Could you check a few things on this model? Use its own coordinates, in mm. A direction names the side the tool comes from. Give positions to 0.01 mm unless a question says otherwise; leave off trailing zeros. Order: outer loops, then holes, each group sorted by start corner. A loop starts at its lowest first (then second) coordinate and runs counter-clockwise, first axis right, second up. Notation, with made-up numbers: M 50,-26 L 109,-26 A14 ccw 109,-14 Z; hole C -15.5,22.5 d1. An arc over 180 degrees is marked long. Use a Markdown table: item, result. Add a question column.
Item 1: If we mould it in two halves opening along Z, with no side actions, what happens to faces 1 (the face through (2.381, 4, -1)), 2 (the face through (3, 6, 2.496)), 3 (the face through (-0.732, 10.339, -2.326))? For each: released by +Z, released by -Z, zero draft, split by the parting line, or undercut.
Item 2: I'm going to push flat-ended pins straight in: pin 1 Ø0.7 at (x, z) = (-1, 3.5) entering from +Y; pin 2 Ø1.5 at (x, z) = (2.5, 3) entering from +Y; pin 3 Ø2.5 at (x, y) = (0, 5.56) entering from -Z; pin 4 Ø1 at (x, y) = (1.5, 6) entering from -Z. Where does each tip first touch, or does it pass through?
Item 3: If I drill on L1, parallel to Y at x = 0, z = 3.55; L2, parallel to X at y = 4, z = -2.25, over which ranges is the centre line in solid material (lowest first)? Write a range as from..to.
Item 4: For faces 4 (the face through (0, 1.778, 3)), 5 (the face through (0, 7.938, -1)), 6 (the face through (0.31, 3.19, 3.22)), 7 (the face through (-2.381, 4, -1)), which set-ups out of +Z, -Z, +X, -X, +Y, -Y let a thin tool reach every point of the face, with its end or its side?
Item 5: Suppose I cut it at A-A on y = 2. Write out the boundary of the cut face in (x, z).
Item 6: Suppose I cut it at D-D on x = 0. Count the separate pieces of the cut face and the enclosed holes in it, plus the area to 3 significant figures.
from build123d import *

# Parameters (mm, degrees)
SKETCH1_W           = 7.9375
SKETCH1_H           = 7.9375
BASE_EXTRUDE_DEPTH  = 9.525
SKETCH2_R           = 2.4384
BOSS_EXTRUDE1_DEPTH = 1.905
SKETCH3_W           = 1.4732
SKETCH3_H           = 7.747
CUT_EXTRUDE1_DEPTH  = 15.470652467
FILLET1_R           = 0.254
SKETCH4_W           = 4.7625
SKETCH4_H           = 4.7625
CUT_EXTRUDE2_DEPTH  = 7.9375
CUT_EXTRUDE3_REACH  = 16.471
SKETCH5_W           = 4.7625
SKETCH5_H           = 4.7625
SKETCH6_R           = 2.3876
BOSS_EXTRUDE2_DEPTH = 1.4732
CUT_EXTRUDE4_REACH  = 16.471
SKETCH7_R           = 1.524


with BuildPart() as part:
    # Sketch1 → Base-Extrude (new body)
    with BuildSketch(Plane(origin=(0, 0, 0), x_dir=(1, 0, 0), z_dir=(0, 1, 0))):
        Rectangle(SKETCH1_W, SKETCH1_H)
    extrude(amount=BASE_EXTRUDE_DEPTH)

    # Sketch2 → Boss-Extrude1 (add)
    with BuildSketch(Plane(origin=(0, 9.525, 0), x_dir=(-1, 0, 0), z_dir=(0, 1, 0))):
        with Locations(Location((0, 0, 0), (0, 0, 270))):
            Circle(SKETCH2_R)
    extrude(amount=BOSS_EXTRUDE1_DEPTH)

    # Sketch3 → Cut-Extrude1 (cut, through all)
    with BuildSketch(Plane(origin=(3.96875, 0, 0), x_dir=(0, 0, -1), z_dir=(1, 0, 0))):
        with Locations((-3.23215, 5.6515)):
            Rectangle(SKETCH3_W, SKETCH3_H)
    extrude(amount=-CUT_EXTRUDE1_DEPTH, mode=Mode.SUBTRACT)

    # Fillet1
    fillet1_edges = [part.edges().sort_by_distance(p)[0] for p in [
        (0, 9.525, -3.96875),
        (0, 11.43, 2.4384),
        (3.96875, 9.525, -0.7366),
        (0, 9.525, 2.49555),
        (-3.96875, 9.525, -0.7366),
    ]]
    fillet(fillet1_edges, radius=FILLET1_R)

    # Sketch4 → Cut-Extrude2 (cut)
    with BuildSketch(Plane.XZ):
        Rectangle(SKETCH4_W, SKETCH4_H)
    extrude(amount=-CUT_EXTRUDE2_DEPTH, mode=Mode.SUBTRACT)

    # Sketch5 → Cut-Extrude3 (cut, up to next)
    with BuildSketch(Plane(origin=(0, 0, -3.96875), x_dir=(-1, 0, 0), z_dir=(0, 0, -1)), mode=Mode.PRIVATE) as cut_extrude3_sk1:
        with Locations((0, 5.55625)):
            Rectangle(SKETCH5_W, SKETCH5_H)
    cut_extrude3_tool1 = extrude(cut_extrude3_sk1.sketch, amount=-CUT_EXTRUDE3_REACH, mode=Mode.PRIVATE) & part.part
    add(cut_extrude3_tool1.solids().sort_by_distance((0, 5.55625, -3.96875))[0], mode=Mode.SUBTRACT)

    # Sketch6 → Boss-Extrude2 (add)
    with BuildSketch(Plane.XY.offset(2.49555)):
        with Locations(Location((0, 5.55625, 0), (0, 0, 180))):
            Circle(SKETCH6_R)
    extrude(amount=BOSS_EXTRUDE2_DEPTH)

    # Sketch7 → Cut-Extrude4 (cut, up to next)
    with BuildSketch(Plane.XY.offset(3.96875), mode=Mode.PRIVATE) as cut_extrude4_sk1:
        with Locations((0, 5.55625)):
            Circle(SKETCH7_R)
    cut_extrude4_tool1 = extrude(cut_extrude4_sk1.sketch, amount=-CUT_EXTRUDE4_REACH, mode=Mode.PRIVATE) & part.part
    add(cut_extrude4_tool1.solids().sort_by_distance((0, 5.55625, 3.96875))[0], mode=Mode.SUBTRACT)


solid = part.part
Findings below:
| question | item | result |
|---|---|---|
| 1 | face 1 | undercut |
| 1 | face 2 | released by +Z |
| 1 | face 3 | split by the parting line |
| 2 | pin 1 | stops at y = 7.85 |
| 2 | pin 2 | stops at y = 9.52 |
| 2 | pin 3 | passes through |
| 2 | pin 4 | stops at z = 2.38 |
| 3 | L1 | y = 0..1.78, 3.17..4.03, 7.08..7.94 |
| 3 | L2 | x = -3.97..-2.38, 2.38..3.97 |
| 4 | face 4 | +Z, +X, -X |
| 4 | face 5 | -Z |
| 4 | face 6 | +Z |
| 4 | face 7 | none |
| 5 | outline | M -3.97,-3.97 L 3.97,-3.97 L 3.97,2.5 L -3.97,2.5 Z; hole M -2.38,-2.38 L 2.38,-2.38 L 2.38,2.38 L -2.38,2.38 Z |
| 6 | separate pieces | 3 |
| 6 | enclosed holes | 0 |
| 6 | area | 30.3 mm^2 |
